Model file for the job. Use its own axes, mm. Face numbers are marked on the shaded views. A direction names the side the tool comes from. Give positions to 0.01 mm unless a question says otherwise; leave off trailing zeros. Loops run counter-clockwise (first coordinate to the right, second up) from the corner with the lowest first, then second, coordinate; pieces in that order, holes last. Notation, with made-up numbers: (-31.75, -19) - (-10.75, -19) arc R25 cw to (-10.75, 7) - close; hole circle Ø1 at (7.25, 23.5). An arc over 180 degrees is marked (long way). Answer as CSV lines item,"result". Start each with the question number.
Item 1: Saw through at A-A on y = -1. Give the cut face in (x, z).
Item 2: Tool access for the marked faces 1, 2 and 3: list every direction of +Z, -Z, +X, -X, +Y, -Y with a clear straight run to the whole face (end or side of a thin tool).
Item 3: Saw through at B-B on x = -31.5. Give the cut face in (y, z), plus the area to 3 significant figures.
Item 4: Drill centre line: L1, parallel to Z at x = 38.5, y = 58. Where is it in solid material? Low to high. Write a range as from..to.
Item 5: Pin check, flat tip, straight feed: pin 1 (12.5 mm diameter, centred on x = 34, y = -34, fed in from +Z). Stop position of the tip, or through.
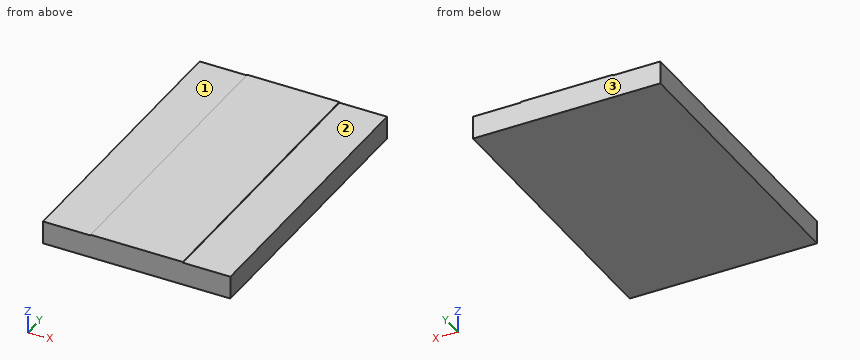
from build123d import *

# Parameters (mm, degrees)
SKETCH1_W           = 100.0125
SKETCH1_H           = 155.575
BOSS_EXTRUDE1_DEPTH = 6.35
CUT_EXTRUDE1_REACH  = 157.575
SKETCH4_W           = 25.4
SKETCH4_H           = 0.396875


with BuildPart() as part:
    # Sketch1 → Boss-Extrude1 (new body, symmetric)
    with BuildSketch(Plane.XY):
        Rectangle(SKETCH1_W, SKETCH1_H)
    extrude(amount=BOSS_EXTRUDE1_DEPTH, both=True)

    # Sketch4 → Cut-Extrude1 (cut, up to next)
    with BuildSketch(Plane(origin=(0, 77.7875, 0), x_dir=(1, 0, 0), z_dir=(0, 1, 0)), mode=Mode.PRIVATE) as cut_extrude1_sk1:
        with Locations((-37.30625, -6.1515625)):
            Rectangle(SKETCH4_W, SKETCH4_H)
    cut_extrude1_tool1 = extrude(cut_extrude1_sk1.sketch, amount=-CUT_EXTRUDE1_REACH, mode=Mode.PRIVATE) & part.part
    add(cut_extrude1_tool1.solids().sort_by_distance((-37.30625, 77.7875, 6.151562))[0], mode=Mode.SUBTRACT)
    # Sketch4 → Cut-Extrude1 (cut, up to next)
    with BuildSketch(Plane(origin=(0, 77.7875, 0), x_dir=(1, 0, 0), z_dir=(0, 1, 0)), mode=Mode.PRIVATE) as cut_extrude1_sk2:
        with Locations((37.30625, -6.1515625)):
            Rectangle(SKETCH4_W, SKETCH4_H)
    cut_extrude1_tool2 = extrude(cut_extrude1_sk2.sketch, amount=-CUT_EXTRUDE1_REACH, mode=Mode.PRIVATE) & part.part
    add(cut_extrude1_tool2.solids().sort_by_distance((37.30625, 77.7875, 6.151563))[0], mode=Mode.SUBTRACT)


solid = part.part
Responses:
1,outline,"(-50.01, -6.35) - (50.01, -6.35) - (50.01, 5.95) - (24.61, 5.95) - (24.61, 6.35) - (-24.61, 6.35) - (-24.61, 5.95) - (-50.01, 5.95) - close"
2,face 1,"+Z, -X, +Y, -Y"
2,face 2,"+Z, +X, +Y, -Y"
2,face 3,"+Z, -Z, +X, -X, +Y"
3,outline,"(-77.79, -6.35) - (77.79, -6.35) - (77.79, 5.95) - (-77.79, 5.95) - close"
3,area,"1,910 mm2"
4,L1,"-6.35..5.95"
5,pin 1,"z = 5.95"
